Geometry: final body of the model. Coordinates: model frame, mm. Face numbers are marked on the shaded views. Give positions to 0.01 mm unless a question says otherwise; leave off trailing zeros. One line per item, written item: value.
```python
from build123d import *

# Parameters (mm, degrees)
F0_W     = 101
F0_H     = 101
F0_W_2   = 42
F0_H_2   = 20
F1_DEPTH = 1
F2_W     = 101
F2_H     = 101
F2_W_2   = 44
F2_H_2   = 22
F3_DEPTH = 100
F4_W     = 15
F4_H     = 90
F5_DEPTH = 101.001


with BuildPart() as f1:
    # F0 (on Top) → F1 (new body)
    with BuildSketch(Plane.XY):
        with Locations((50.5, 50.5)):
            Rectangle(F0_W, F0_H)
        with Locations((26, 15)):
            Rectangle(F0_W_2, F0_H_2, mode=Mode.SUBTRACT)
        with Locations((26, 39)):
            Rectangle(F0_W_2, F0_H_2, mode=Mode.SUBTRACT)
        with Locations((75, 15)):
            Rectangle(F0_W_2, F0_H_2, mode=Mode.SUBTRACT)
        with Locations((75, 39)):
            Rectangle(F0_W_2, F0_H_2, mode=Mode.SUBTRACT)
        with Locations((26, 63)):
            Rectangle(F0_W_2, F0_H_2, mode=Mode.SUBTRACT)
        with Locations((26, 87)):
            Rectangle(F0_W_2, F0_H_2, mode=Mode.SUBTRACT)
        with Locations((75, 63)):
            Rectangle(F0_W_2, F0_H_2, mode=Mode.SUBTRACT)
        with Locations((75, 87)):
            Rectangle(F0_W_2, F0_H_2, mode=Mode.SUBTRACT)
    extrude(amount=F1_DEPTH)

    # F2 (on face) → F3 (join)
    with BuildSketch(Plane.XY.offset(1)):
        with Locations((50.5, 50.5)):
            Rectangle(F2_W, F2_H)
        with Locations((26, 15)):
            Rectangle(F2_W_2, F2_H_2, mode=Mode.SUBTRACT)
        with Locations((26, 39)):
            Rectangle(F2_W_2, F2_H_2, mode=Mode.SUBTRACT)
        with Locations((75, 15)):
            Rectangle(F2_W_2, F2_H_2, mode=Mode.SUBTRACT)
        with Locations((75, 39)):
            Rectangle(F2_W_2, F2_H_2, mode=Mode.SUBTRACT)
        with Locations((26, 63)):
            Rectangle(F2_W_2, F2_H_2, mode=Mode.SUBTRACT)
        with Locations((26, 87)):
            Rectangle(F2_W_2, F2_H_2, mode=Mode.SUBTRACT)
        with Locations((75, 63)):
            Rectangle(F2_W_2, F2_H_2, mode=Mode.SUBTRACT)
        with Locations((75, 87)):
            Rectangle(F2_W_2, F2_H_2, mode=Mode.SUBTRACT)
    extrude(amount=F3_DEPTH)

    # F4 (on face) → F5 (cut, through all)
    with BuildSketch(Plane(origin=(0, 0, 0), x_dir=(0, -1, 0), z_dir=(-1, 0, 0))):
        with Locations((-88.5, 51)):
            Rectangle(F4_W, F4_H)
        with Locations((-63.5, 51)):
            Rectangle(F4_W, F4_H)
        with Locations((-38.5, 51)):
            Rectangle(F4_W, F4_H)
        with Locations((-13.5, 51)):
            Rectangle(F4_W, F4_H)
    extrude(amount=-F5_DEPTH, mode=Mode.SUBTRACT)


solid = f1.part
```
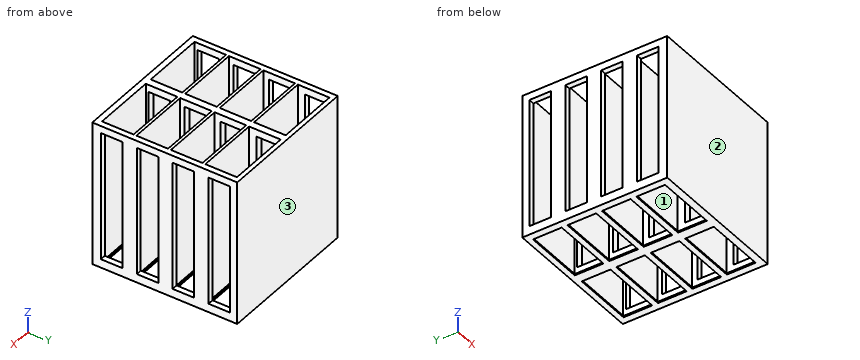
1) Mould query, pull axis Y, two halves, no side actions, for the marked faces 1, 2 and 3. Classes: released by +Y, released by -Y, zero draft, split by the parting line, or undercut.
Answers below:
face 1: undercut
face 2: released by -Y
face 3: released by +Y
2) Material intervals for line 1 along Y through (x, z) = (32, 16.5); line 2 along X through (y, z) = (79.5, 74.5); line 3 along Z through (x, y) = (49, 69), sorted ascending.
Answers below:
line 1: 0 to 4, 26 to 28, 50 to 52, 74 to 76, 98 to 101
line 2: 0 to 4, 48 to 53, 97 to 101
line 3: 0 to 6, 96 to 101
3) Section A-A, the plane y = 17.5. Count the separate pieces of the cut face and the enclosed holes in it, then the cut area to 3 significant figures.
Answers below:
separate pieces: 6
enclosed holes: 0
area: 147 mm^2
